The drawing under review shows one solid part. Ordinate dimensions are in mm from its lowest x, y, z. Give positions to 0.01 mm unless a question says otherwise; leave off trailing zeros. Write each loop counter-clockwise with the first axis right and the second up, starting at its lowest first coordinate (ties: lowest second). Pieces come first, ordered by that corner, then holes. Notation, with made-up numbers: (71.5, -31.5) - (90.5, -31.5) arc R9 ccw to (90.5, -22.5) - close; hole circle Ø3 at (73, 50.5). An arc over 180 degrees is marked (long way). Write item = value, one per line.
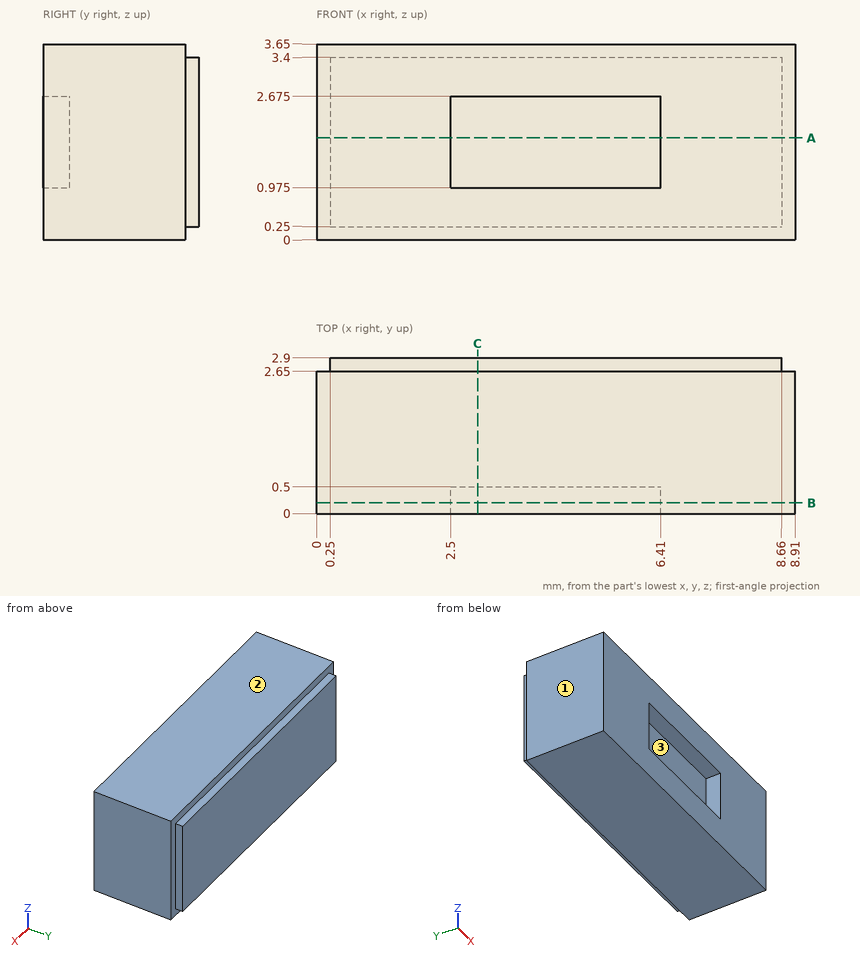
1. Take a section at C-C on x = 3. Give the boundary of the cut face in (y, z) (3 decimals), and give its area (3 significant figures).
Findings below:
outline = (0, 0) - (2.65, 0) - (2.65, 0.25) - (2.9, 0.25) - (2.9, 3.4) - (2.65, 3.4) - (2.65, 3.65) - (0, 3.65) - (0, 2.675) - (0.5, 2.675) - (0.5, 0.975) - (0, 0.975) - close
area = 9.61 mm²
2. For line 1 (X direction, y = 0.2, z = 2); line 2 (Y direction, x = 2.75, z = 1.65); line 3 (Z direction, x = 3.75, y = 2.75), list the stretches that pass through material, from the lowest coordinate up. Write a range as from..to.
Findings below:
line_1 = 0..2.5, 6.41..8.91
line_2 = 0.5..2.9
line_3 = 0.25..3.4
3. Take a section at B-B on y = 0.2. Give the boundary of the cut face in (x, z) (3 decimals).
Findings below:
outline = (0, 0) - (8.91, 0) - (8.91, 3.65) - (0, 3.65) - close; hole (2.5, 0.975) - (6.41, 0.975) - (6.41, 2.675) - (2.5, 2.675) - close
4. Draft analysis for pull direction X (two halves, no side actions). For the marked faces 1, 2 and 3, state which applies: +X half, -X half, draft (parallel to the pull), parting line (faces both ways), or undercut.
Findings below:
face_1 = -X half
face_2 = draft
face_3 = undercut
5. Take a section at A-A on z = 1.9. Give the boundary of the cut face in (x, y).
Findings below:
outline = (0, 0) - (2.5, 0) - (2.5, 0.5) - (6.41, 0.5) - (6.41, 0) - (8.91, 0) - (8.91, 2.65) - (8.66, 2.65) - (8.66, 2.9) - (0.25, 2.9) - (0.25, 2.65) - (0, 2.65) - close
